Here's the drawing with two shaded views (mm, measured from the low corner). I have some questions. A direction names the side the tool comes from. Give positions to 0.01 mm unless a question says otherwise; leave off trailing zeros. Loops run counter-clockwise (first coordinate to the right, second up) from the corner with the lowest first, then second, coordinate; pieces in that order, holes last.
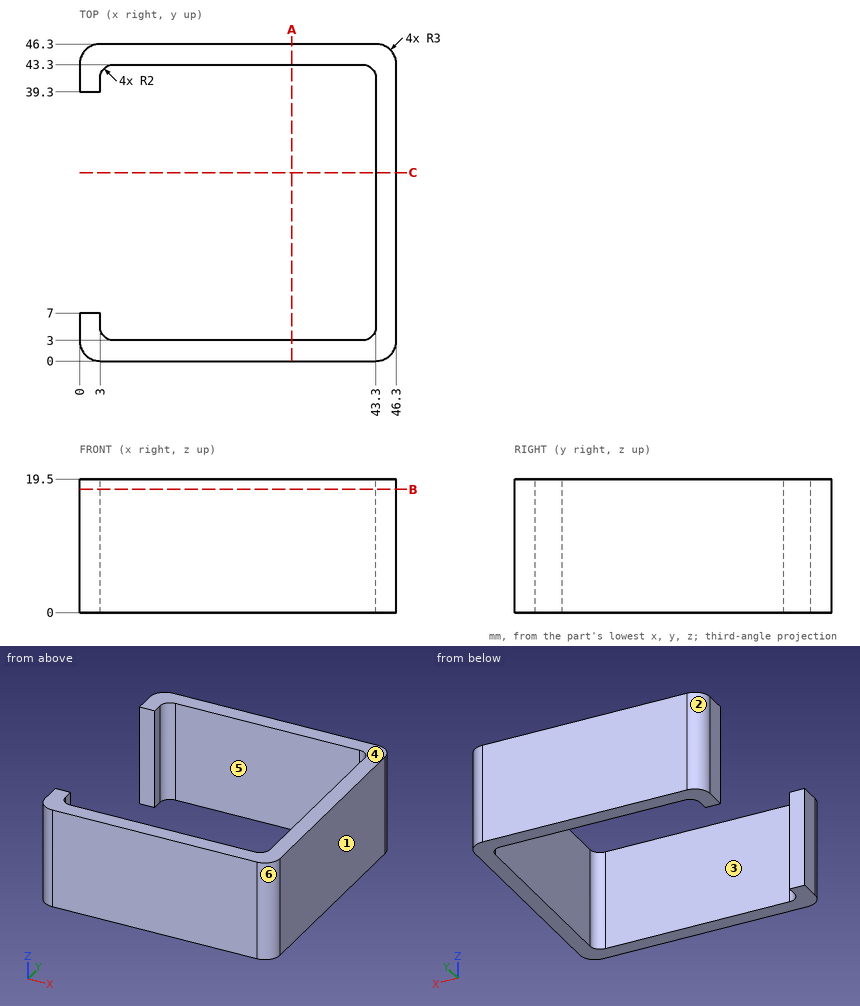
(1) Will these pins go through, and if not, where does the flat tip stop? P1, Ø4, axis at y = 23, z = 12.5, coming from the -X side; P2, Ø3.5, axis at x = 1, z = 14, coming from the -Y side.
Returned:
P1: stops at x = 43.3
P2: stops at y = 0.01
(2) Suppose I cut it at A-A on x = 31. List the corners of the cut face in (y, z) for me, plus the area to 3 significant figures.
Returned:
outline: (0, 0) - (3, 0) - (3, 19.5) - (0, 19.5) - close; (43.3, 0) - (46.3, 0) - (46.3, 19.5) - (43.3, 19.5) - close
area: 117 mm2
(3) Which directions (+Z, -Z, +X, -X, +Y, -Y) give clear straight access to the entire face, cutting with the end or side of a thin tool? Please do the marked faces 5 and 6.
Returned:
face 5: +Z, -Z
face 6: +Z, -Z, +X, -Y
(4) Thinking about a two-plate mould opening in X: for the marked faces 1, 2, 3 and 4, which applies, pulls with the +X half, pulls with the -X half, needs draft (parallel to the pull), parting line crosses it, or undercut?
Returned:
face 1: pulls with the +X half
face 2: pulls with the -X half
face 3: undercut
face 4: needs draft
(5) Please list where these lines run through material, in increasing order: probe 1 along Y at (x, z) = (12.5, 17); probe 2 along X at (y, z) = (28.5, 6.75).
Returned:
probe 1: y = 0 to 3, 43.3 to 46.3
probe 2: x = 43.3 to 46.3
(6) Suppose I cut it at B-B on z = 18. List the corners of the cut face in (x, y) for me, plus the area to 3 significant figures.
Returned:
outline: (0, 3) arc R3 ccw to (3, 0) - (43.3, 0) arc R3 ccw to (46.3, 3) - (46.3, 43.3) arc R3 ccw to (43.3, 46.3) - (3, 46.3) arc R3 ccw to (0, 43.3) - (0, 39.3) - (3, 39.3) - (3, 41.3) arc R2 cw to (5, 43.3) - (41.3, 43.3) arc R2 cw to (43.3, 41.3) - (43.3, 5) arc R2 cw to (41.3, 3) - (5, 3) arc R2 cw to (3, 5) - (3, 7) - (0, 7) - close
area: 418 mm2
(7) Suppose I cut it at C-C on y = 27.5. List the corners of the cut face in (x, z) for me, plus the area to 3 significant figures.
Returned:
outline: (43.3, 0) - (46.3, 0) - (46.3, 19.5) - (43.3, 19.5) - close
area: 58.5 mm2
